```python
from build123d import *

# Parameters (mm, degrees)
F0_R     = 550
F0_R_2   = 60
F1_DEPTH = 25
F2_R     = 225
F2_R_2   = 200
F3_DEPTH = 950
F4_R     = 350
F4_R_2   = 225
F4_R_3   = 200
F4_R_4   = 60
F5_DEPTH = 25


with BuildPart() as f1:
    # F0 (on Top) → F1 (new body)
    with BuildSketch(Plane.XY):
        Circle(F0_R)
        Circle(F0_R_2, mode=Mode.SUBTRACT)
    extrude(amount=-F1_DEPTH)

    # F2 (on face) → F3 (join)
    with BuildSketch(Plane(origin=(0, 0, -25), x_dir=(1, 0, 0), z_dir=(0, 0, -1))):
        Circle(F2_R)
        Circle(F2_R_2, mode=Mode.SUBTRACT)
    extrude(amount=F3_DEPTH)

    # F4 (on face) → F5 (join)
    with BuildSketch(Plane(origin=(0, 0, -975), x_dir=(1, 0, 0), z_dir=(0, 0, -1))):
        Circle(F4_R)
        Circle(F4_R_2, mode=Mode.SUBTRACT)
        Circle(F4_R_2)
        Circle(F4_R_3, mode=Mode.SUBTRACT)
        Circle(F4_R_3)
        Circle(F4_R_4, mode=Mode.SUBTRACT)
    extrude(amount=F5_DEPTH)


solid = f1.part
```
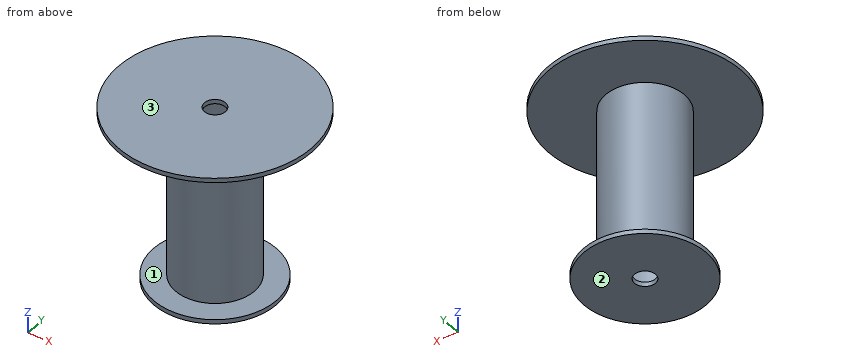
Model file for the job. Use its own axes, mm. Face numbers are marked on the shaded views. Give positions to 0.01 mm unless a question says otherwise; leave off trailing zeros. Write each loop counter-clockwise with the first axis right and the second up, starting at its lowest first coordinate (ties: lowest second). Pieces come first, ordered by that corner, then holes. Notation, with made-up numbers: (-9.5, -12.75) -> (3.5, -12.75) arc R7 cw to (3.5, 0.25) -> close; hole circle Ø3 at (72, 78.25). An arc over 180 degrees is marked (long way). Use CSV: the item, a comma, the result in double quotes. Start each with the question number.
1) Two-plate mould, pull along Z, no slides. Class the marked faces 1, 2 and 3: released by +Z, released by -Z, zero draft, split by the parting line, or undercut.
2) Cut at C-C on z = -198.5. List the corners of the cut face in (x, y), plus the area to 3 significant figures.
3) Drill centre lines: L1, parallel to Z at x = -25, y = 246; L2, parallel to X at y = 0, z = -367; L3, parallel to Y at x = 3.5, z = -182. Where is each one in solid material? Low to high.
4) Cut at A-A on x = 0. List the corners of the cut face in (y, z).
5) Pin check, flat tips, straight feed: P1, Ø5, axis at y = -121.5, z = -516.5, coming from the +X side; P2, Ø4, axis at x = 48, z = -356.5, coming from the +Y side; P3, Ø2, axis at y = 203.5, z = -357, coming from the +X side. Stop position of each tip, or through.
6) Cut at D-D on y = -117.5. List the corners of the cut face in (x, z).
Final values:
1,face 1,"undercut"
1,face 2,"released by -Z"
1,face 3,"released by +Z"
2,outline,"circle Ø450 at (0, 0); hole circle Ø400 at (0, 0)"
2,area,"33,400 mm2"
3,L1,"z = -1000 to -975, -25 to 0"
3,L2,"x = -225 to -200, 200 to 225"
3,L3,"y = -224.97 to -199.97, 199.97 to 224.97"
4,outline,"(-550, -25) -> (-225, -25) -> (-225, -975) -> (-350, -975) -> (-350, -1000) -> (-60, -1000) -> (-60, -975) -> (-200, -975) -> (-200, -25) -> (-60, -25) -> (-60, 0) -> (-550, 0) -> close; (60, -1000) -> (350, -1000) -> (350, -975) -> (225, -975) -> (225, -25) -> (550, -25) -> (550, 0) -> (60, 0) -> (60, -25) -> (200, -25) -> (200, -975) -> (60, -975) -> close"
5,P1,"stops at x = 190.96"
5,P2,"stops at y = 220.25"
5,P3,"stops at x = 98.08"
6,outline,"(-537.3, -25) -> (-191.88, -25) -> (-191.88, -975) -> (-329.69, -975) -> (-329.69, -1000) -> (329.69, -1000) -> (329.69, -975) -> (191.88, -975) -> (191.88, -25) -> (537.3, -25) -> (537.3, 0) -> (-537.3, 0) -> close; hole (-161.84, -975) -> (161.84, -975) -> (161.84, -25) -> (-161.84, -25) -> close"
